Solid Edge part; units mm, degrees
sketch "Sketch1" plane through (0, 0, 0) normal (0, -1, 0) x (1, 0, 0)
  circle A0 centre (0, 0) radius 30
extrude "Protrusion1" add sketch "Sketch1" against normal blind 275
sketch "Sketch2" plane through (0, 0, 0) normal (0, -1, 0) x (1, 0, 0)
  circle A0 centre (0, 0) radius 45
extrude "ExtrudedProtrusion_2" add sketch "Sketch2" against normal blind 10
mirror "Mirror1" about plane through (0, 137.5, 0) normal (0, -1, 0) of "ExtrudedProtrusion_2"
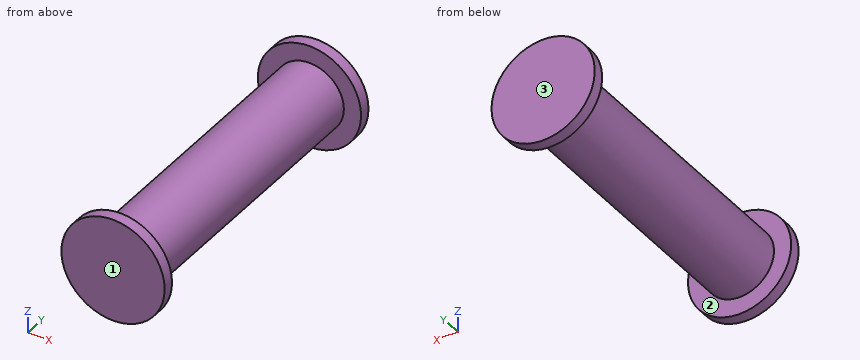
CAD build for the part. Positions are in the model's coordinates, mm. Face numbers are marked on the shaded views. Give positions to 0.01 mm unless a question says otherwise; leave off trailing zeros. Loops run counter-clockwise (first coordinate to the right, second up) from the corner with the lowest first, then second, coordinate; pieces in that order, holes last. Notation, with made-up numbers: M -8,30.5 L 10,30.5 A22 ccw 10,68.5 Z; hole C 20,33.25 d3. An arc over 180 degrees is marked long. Use one line per item in the form item = value.
Item 1: Drill centre lines: probe 1 along Y at (x, z) = (31, -1.5); probe 2 along X at (y, z) = (83, -1.5); probe 3 along Z at (x, y) = (-6.5, 85). Where is each one in solid material? Low to high. Write a range as from..to.
Determined:
probe_1 = 0..10, 265..275
probe_2 = -29.96..29.96
probe_3 = -29.29..29.29
Item 2: Flat gauge pins, fed straight in: pin 1 (12 mm diameter, centred on y = 130.5, z = 29, fed in from -X); pin 2 (8 mm diameter, centred on y = 131, z = -26.5, fed in from +X); pin 3 (5 mm diameter, centred on x = 9.5, y = 66.5, fed in from +Z). Where does each tip first touch, or does it go through?
Determined:
pin_1 = -19.26
pin_2 = 19.84
pin_3 = 29.17
Item 3: Slice it at C-C (y = 36). List the corners of the cut face in (x, z), plus the area to 3 significant figures.
Determined:
outline = C 0,0 d60
area = 2,830 mm2
Item 4: Two-plate mould, pull along Y, no slides. Class the marked faces 1, 2 and 3: pulls with the +Y half, pulls with the -Y half, needs draft (parallel to the pull), parting line crosses it, or undercut.
Determined:
face_1 = pulls with the -Y half
face_2 = undercut
face_3 = pulls with the +Y half
Item 5: Slice it at A-A (z = 0). List the corners of the cut face in (x, y), plus the area to 3 significant figures.
Determined:
outline = M -45,0 L 45,0 L 45,10 L 30,10 L 30,265 L 45,265 L 45,275 L -45,275 L -45,265 L -30,265 L -30,10 L -45,10 Z
area = 17,100 mm2
Item 6: Slice it at B-B (x = 0). List the corners of the cut face in (y, z).
Determined:
outline = M 0,-45 L 10,-45 L 10,-30 L 265,-30 L 265,-45 L 275,-45 L 275,45 L 265,45 L 265,30 L 10,30 L 10,45 L 0,45 Z
